Can you work these out from the model? Positions are in its coordinate system, mm. Face numbers are marked on the shaded views. A direction names the side the tool comes from. Give positions to 0.01 mm unless a question says otherwise; leave off trailing zeros. Write each loop counter-clockwise with the first axis right and the second up, starting at its lowest first coordinate (ties: lowest second). Pieces come first, ordered by that corner, then holes.
Autodesk Inventor part; units mm, degrees
ref_plane "Plan YZ" through (0, 0, 0) normal (1, 0, 0) x (0, 1, 0)
ref_plane "Plan XZ" through (0, 0, 0) normal (0, 1, 0) x (-1, 0, 0)
ref_plane "Plan XY" through (0, 0, 0) normal (0, 0, 1) x (1, 0, 0)
sketch "Esquisse1" plane through (0, 0, 0) normal (0, 0, 1) x (1, 0, 0)
  circle A0 centre (0, 0) radius 25
  arc A1 (4, 2.1685) -> (-4, 2.1685) centre (0, 0) ccw
  line L0 (-4, -2.1685) -> (-4, 2.1685)
  arc A2 (-4, -2.1685) -> (4, -2.1685) centre (0, 0) ccw
  line L1 (4, -2.1685) -> (4, 2.1685)
  line L2 (0, -35) -> (0, 35) construction
  line L3 (-35, 0) -> (35, 0) construction
  point P0 (0, 0)
  dimension "d0" = 50
  dimension "d1" = 8
  dimension "d2" = 4.55
extrude "Extrusion1" add sketch "Esquisse1" along normal blind 3
sketch "Esquisse6" plane through (0, 0, 3) normal (0, 0, 1) x (1, 0, 0)
  line L0 (-35, 0) -> (35, 0) construction
  line L1 (0, -35) -> (0, 35) construction
  circle A0 centre (0, 0) radius 18.5 construction
  point P0 (-18.5, 0)
  point P1 (15.5644, -10)
  point P2 (15.5644, 10)
  dimension "d5" = 37
  dimension "d6" = 20
hole "Perçage1" at (-18.5, 0, 3) at (15.5644, -10, 3) at (15.5644, 10, 3) direction (0, 0, -1) diameter 2.459 end through all
properties part number "Couvercle_haut" material "Plastique PMMA"
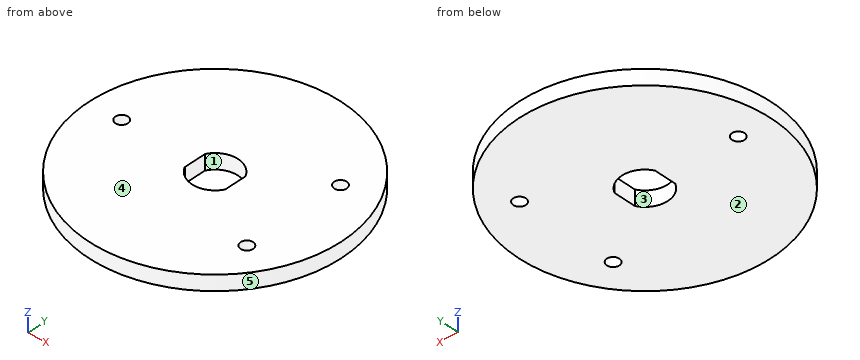
(1) If I drill on L1, parallel to X at y = -0.5, z = 2.2 (3 decimals); L2, parallel to X at y = -10, z = 1.6; L3, parallel to Y at x = -18.5, z = 2, over which ranges is the centre line in solid material (lowest first)?
Returned:
L1: x = -24.995 to -19.623, -17.377 to -4, 4 to 24.995
L2: x = -22.91 to 14.33, 16.79 to 22.91
L3: y = -16.82 to -1.23, 1.23 to 16.82
(2) Imagine slicing it at C-C, the plane y = 10. Write out the boundary of the cut face in (x, z).
Returned:
outline: (-22.91, 0) - (14.33, 0) - (14.33, 3) - (-22.91, 3) - close; (16.79, 0) - (22.91, 0) - (22.91, 3) - (16.79, 3) - close
(3) For the marked faces 1 and 2, which set-ups out of +Z, -Z, +X, -X, +Y, -Y let a thin tool reach every point of the face, with its end or its side?
Returned:
face 1: +Z, -Z
face 2: -Z, +X, -X, +Y, -Y
(4) Will these pins go through, and if not, where does the flat tip stop? P1, Ø1.5, axis at x = 15.56, y = -10, coming from the -Z side; P2, Ø1, axis at y = -14.5, z = 1, coming from the +X side.
Returned:
P1: passes through
P2: stops at x = 20.71
(5) Imagine slicing it at A-A, the plane y = 0. Write out the boundary of the cut face in (x, z), plus the area to 3 significant figures.
Returned:
outline: (-25, 0) - (-19.73, 0) - (-19.73, 3) - (-25, 3) - close; (-17.27, 0) - (-4, 0) - (-4, 3) - (-17.27, 3) - close; (4, 0) - (25, 0) - (25, 3) - (4, 3) - close
area: 119 mm2
(6) If we mould it in two halves opening along Y, with no side actions, what happens to the marked faces 3, 4 and 5? For each: +Y half, -Y half, draft (parallel to the pull), parting line (faces both ways), or undercut.
Returned:
face 3: undercut
face 4: draft
face 5: parting line
(7) Imagine slicing it at B-B, the plane x = 0. Write out the boundary of the cut face in (y, z), plus the area to 3 significant figures.
Returned:
outline: (-25, 0) - (-4.55, 0) - (-4.55, 3) - (-25, 3) - close; (4.55, 0) - (25, 0) - (25, 3) - (4.55, 3) - close
area: 123 mm2
(8) Imagine slicing it at D-D, the plane z = 1.45. Write out the boundary of the cut face in (x, y), plus the area to 3 significant figures.
Returned:
outline: circle Ø50 at (0, 0); hole circle Ø2.46 at (-18.5, 0); hole (-4, -2.17) arc R4.55 ccw to (4, -2.17) - (4, 2.17) arc R4.55 ccw to (-4, 2.17) - close; hole circle Ø2.46 at (15.56, -10); hole circle Ø2.46 at (15.56, 10)
area: 1,890 mm2
